Verification items for the finished model (mm, model axes). Face numbers are marked on the shaded views. A direction names the side the tool comes from. Give positions to 0.01 mm unless a question says otherwise; leave off trailing zeros. Write each loop counter-clockwise with the first axis right and the second up, starting at its lowest first coordinate (ties: lowest second). Pieces come first, ordered by that corner, then holes. Notation, with made-up numbers: (-11, -5.75) -> (19, -5.75) arc R22 ccw to (19, 33.25) -> close; hole circle Ø6 at (70, -11.5). An arc over 180 degrees is marked (long way). Use CSV: the item, a comma, the result in double quotes. Start each with the question number.
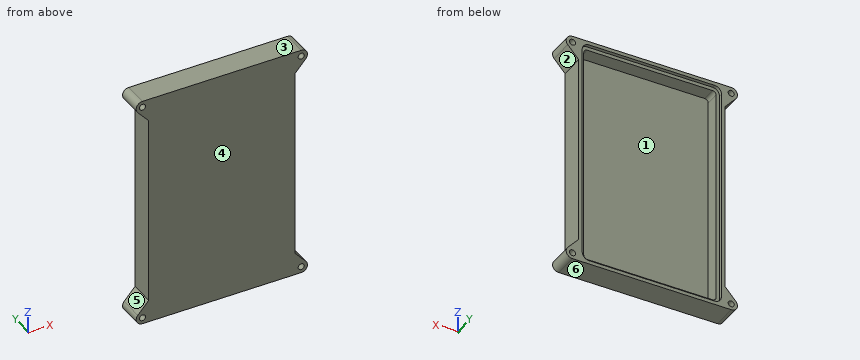
```python
from build123d import *

# Parameters (mm, degrees)
SALIENTE_EXTRUIR2_DEPTH   = 11
SALIENTE_EXTRUIR3_DEPTH   = 25.5
SALIENTE_EXTRUIR4_DEPTH   = 2.5
SALIENTE_EXTRUIR5_DEPTH   = 36.5
SIMETR_A2_COPY_1_DEPTH    = 36.5
CROQUIS6_R                = 2.2
CORTAR_EXTRUIR2_DEPTH     = 112.083302076
SIMETR_A4_COPY_1_SKETCH_R = 2.2
SIMETR_A4_COPY_1_DEPTH    = 112.083302076
CORTAR_EXTRUIR3_DEPTH     = 6
CORTAR_EXTRUIR4_START     = -18
CORTAR_EXTRUIR4_DEPTH     = 18
CORTAR_EXTRUIR5_START     = -13
CORTAR_EXTRUIR5_DEPTH     = 13


with BuildPart() as part:
    # Croquis1 → Saliente-Extruir2 (new body)
    # profile 1 of 3: a face of its own
    with BuildSketch(Plane(origin=(0, 0, 0), x_dir=(1, 0, 0), z_dir=(0, 1, 0))):
        with BuildLine():
            Line((-45, 85), (45, 85))
            ThreePointArc((45, 85), (50.303300859, 82.803300859), (52.5, 77.5))
            Line((52.5, 77.5), (52.5, -77.5))
            ThreePointArc((52.5, -77.5), (50.303300859, -82.803300859), (45, -85))
            Line((45, -85), (-45, -85))
            ThreePointArc((-45, -85), (-50.303300859, -82.803300859), (-52.5, -77.5))
            Line((-52.5, -77.5), (-52.5, 77.5))
            ThreePointArc((-52.5, 77.5), (-50.303300859, 82.803300859), (-45, 85))
        make_face()
        with BuildLine():
            ThreePointArc((-45, 82.5), (-48.535533906, 81.035533906), (-50, 77.5))
            Line((-50, 77.5), (-50, -77.5))
            ThreePointArc((-50, -77.5), (-48.535533906, -81.035533906), (-45, -82.5))
            Line((-45, -82.5), (45, -82.5))
            ThreePointArc((45, -82.5), (48.535533906, -81.035533906), (50, -77.5))
            Line((50, -77.5), (50, 77.5))
            ThreePointArc((50, 77.5), (48.535533906, 81.035533906), (45, 82.5))
            Line((45, 82.5), (-45, 82.5))
        make_face(mode=Mode.SUBTRACT)
    # profile 2 of 3: a face of its own
    with BuildSketch(Plane(origin=(0, 0, 0), x_dir=(1, 0, 0), z_dir=(0, 1, 0))):
        with BuildLine():
            Line((-45, 82.5), (45, 82.5))
            ThreePointArc((45, 82.5), (48.535533906, 81.035533906), (50, 77.5))
            Line((50, 77.5), (50, -77.5))
            ThreePointArc((50, -77.5), (48.535533906, -81.035533906), (45, -82.5))
            Line((45, -82.5), (-45, -82.5))
            ThreePointArc((-45, -82.5), (-48.535533906, -81.035533906), (-50, -77.5))
            Line((-50, -77.5), (-50, 77.5))
            ThreePointArc((-50, 77.5), (-48.535533906, 81.035533906), (-45, 82.5))
        make_face()
        with BuildLine():
            ThreePointArc((45, -80), (46.767766953, -79.267766953), (47.5, -77.5))
            Line((47.5, -77.5), (47.5, 77.5))
            ThreePointArc((47.5, 77.5), (46.767766953, 79.267766953), (45, 80))
            Line((45, 80), (-45, 80))
            ThreePointArc((-45, 80), (-46.767766953, 79.267766953), (-47.5, 77.5))
            Line((-47.5, 77.5), (-47.5, -77.5))
            ThreePointArc((-47.5, -77.5), (-46.767766953, -79.267766953), (-45, -80))
            Line((-45, -80), (45, -80))
        make_face(mode=Mode.SUBTRACT)
    # profile 3 of 3: a face of its own
    with BuildSketch(Plane(origin=(0, 0, 0), x_dir=(1, 0, 0), z_dir=(0, 1, 0))):
        with BuildLine():
            Line((-45, -80), (45, -80))
            ThreePointArc((45, -80), (46.767766953, -79.267766953), (47.5, -77.5))
            Line((47.5, -77.5), (47.5, 77.5))
            ThreePointArc((47.5, 77.5), (46.767766953, 79.267766953), (45, 80))
            Line((45, 80), (-45, 80))
            ThreePointArc((-45, 80), (-46.767766953, 79.267766953), (-47.5, 77.5))
            Line((-47.5, 77.5), (-47.5, -77.5))
            ThreePointArc((-47.5, -77.5), (-46.767766953, -79.267766953), (-45, -80))
        make_face()
    extrude(amount=SALIENTE_EXTRUIR2_DEPTH)

    # Croquis2 → Saliente-Extruir3 (add)
    # profile 1 of 2: a face of its own
    with BuildSketch(Plane(origin=(0, 11, 0), x_dir=(1, 0, 0), z_dir=(0, 1, 0))):
        with BuildLine():
            ThreePointArc((52.5, 77.5), (50.303300859, 82.803300859), (45, 85))
            Line((45, 85), (-45, 85))
            ThreePointArc((-45, 85), (-50.303300859, 82.803300859), (-52.5, 77.5))
            Line((-52.5, 77.5), (-52.5, -77.5))
            ThreePointArc((-52.5, -77.5), (-50.303300859, -82.803300859), (-45, -85))
            Line((-45, -85), (45, -85))
            ThreePointArc((45, -85), (50.303300859, -82.803300859), (52.5, -77.5))
            Line((52.5, -77.5), (52.5, 77.5))
        make_face()
        with BuildLine():
            ThreePointArc((-45, 82.5), (-48.535533906, 81.035533906), (-50, 77.5))
            Line((-50, 77.5), (-50, -77.5))
            ThreePointArc((-50, -77.5), (-48.535533906, -81.035533906), (-45, -82.5))
            Line((-45, -82.5), (45, -82.5))
            ThreePointArc((45, -82.5), (48.535533906, -81.035533906), (50, -77.5))
            Line((50, -77.5), (50, 77.5))
            ThreePointArc((50, 77.5), (48.535533906, 81.035533906), (45, 82.5))
            Line((45, 82.5), (-45, 82.5))
        make_face(mode=Mode.SUBTRACT)
    # profile 2 of 2: a face of its own
    with BuildSketch(Plane(origin=(0, 11, 0), x_dir=(1, 0, 0), z_dir=(0, 1, 0))):
        with BuildLine():
            Line((45, 82.5), (-45, 82.5))
            ThreePointArc((-45, 82.5), (-48.535533906, 81.035533906), (-50, 77.5))
            Line((-50, 77.5), (-50, -77.5))
            ThreePointArc((-50, -77.5), (-48.535533906, -81.035533906), (-45, -82.5))
            Line((-45, -82.5), (45, -82.5))
            ThreePointArc((45, -82.5), (48.535533906, -81.035533906), (50, -77.5))
            Line((50, -77.5), (50, 77.5))
            ThreePointArc((50, 77.5), (48.535533906, 81.035533906), (45, 82.5))
        make_face()
        with BuildLine():
            ThreePointArc((-45, 80), (-46.767766953, 79.267766953), (-47.5, 77.5))
            Line((-47.5, 77.5), (-47.5, -77.5))
            ThreePointArc((-47.5, -77.5), (-46.767766953, -79.267766953), (-45, -80))
            Line((-45, -80), (45, -80))
            ThreePointArc((45, -80), (46.767766953, -79.267766953), (47.5, -77.5))
            Line((47.5, -77.5), (47.5, 77.5))
            ThreePointArc((47.5, 77.5), (46.767766953, 79.267766953), (45, 80))
            Line((45, 80), (-45, 80))
        make_face(mode=Mode.SUBTRACT)
    extrude(amount=SALIENTE_EXTRUIR3_DEPTH)

    # Croquis3 → Saliente-Extruir4 (add)
    with BuildSketch(Plane(origin=(0, 36.5, 0), x_dir=(1, 0, 0), z_dir=(0, 1, 0))):
        with BuildLine():
            Line((45, 82.5), (-45, 82.5))
            ThreePointArc((-45, 82.5), (-48.535533906, 81.035533906), (-50, 77.5))
            Line((-50, 77.5), (-50, -77.5))
            ThreePointArc((-50, -77.5), (-48.535533906, -81.035533906), (-45, -82.5))
            Line((-45, -82.5), (45, -82.5))
            ThreePointArc((45, -82.5), (48.535533906, -81.035533906), (50, -77.5))
            Line((50, -77.5), (50, 77.5))
            ThreePointArc((50, 77.5), (48.535533906, 81.035533906), (45, 82.5))
        make_face()
        with BuildLine():
            Line((-47.5, -77.5), (-47.5, 77.5))
            ThreePointArc((-47.5, 77.5), (-46.767766953, 79.267766953), (-45, 80))
            Line((-45, 80), (45, 80))
            ThreePointArc((45, 80), (46.767766953, 79.267766953), (47.5, 77.5))
            Line((47.5, 77.5), (47.5, -77.5))
            ThreePointArc((47.5, -77.5), (46.767766953, -79.267766953), (45, -80))
            Line((45, -80), (-45, -80))
            ThreePointArc((-45, -80), (-46.767766953, -79.267766953), (-47.5, -77.5))
        make_face(mode=Mode.SUBTRACT)
    extrude(amount=SALIENTE_EXTRUIR4_DEPTH)

    # Croquis4 → Saliente-Extruir5 (add)
    with BuildSketch(Plane.XZ):
        with BuildLine():
            Line((57, 85), (45, 85))
            ThreePointArc((45, 85), (50.303300859, 82.803300859), (52.5, 77.5))
            Line((52.5, 77.5), (52.5, 68.686877301))
            Line((52.5, 68.686877301), (60.359510947, 77.506058418))
            ThreePointArc((60.359510947, 77.506058418), (61.10625968, 82.340823577), (57, 85))
        make_face()
    saliente_extruir5 = extrude(amount=-SALIENTE_EXTRUIR5_DEPTH)

    # Simetría1: Saliente-Extruir5 across plane
    add(saliente_extruir5.mirror(Plane(origin=(0, 0, 0), x_dir=(0, 0, 1), z_dir=(1, 0, 0))))

    # Simetría2: Saliente-Extruir5 across plane
    add(saliente_extruir5.mirror(Plane.XY))

    # Simetría2 copy 1 sketch → Simetría2 copy 1 (add)
    with BuildSketch(Plane(origin=(0, 0, 0), x_dir=(-1, 0, 0), z_dir=(0, -1, 0))):
        with BuildLine():
            Line((57, 85), (45, 85))
            ThreePointArc((45, 85), (50.303300859, 82.803300859), (52.5, 77.5))
            Line((52.5, 77.5), (52.5, 68.686877301))
            Line((52.5, 68.686877301), (60.359510947, 77.506058418))
            ThreePointArc((60.359510947, 77.506058418), (61.10625968, 82.340823577), (57, 85))
        make_face()
    extrude(amount=-SIMETR_A2_COPY_1_DEPTH)

    # Croquis6 → Cortar-Extruir2 (cut, through all)
    with BuildSketch(Plane(origin=(0, 36.5, 0), x_dir=(1, 0, 0), z_dir=(0, 1, 0))):
        with Locations(Location((57, 80.5, 0), (0, 0, 270))):
            Circle(CROQUIS6_R)
    cortar_extruir2 = extrude(amount=-CORTAR_EXTRUIR2_DEPTH, mode=Mode.SUBTRACT)

    # Simetría3: Cortar-Extruir2 across plane
    add(cortar_extruir2.mirror(Plane(origin=(0, 0, 0), x_dir=(0, 0, 1), z_dir=(1, 0, 0))), mode=Mode.SUBTRACT)

    # Simetría4: Cortar-Extruir2 across plane
    add(cortar_extruir2.mirror(Plane.XY), mode=Mode.SUBTRACT)

    # Simetría4 copy 1 sketch → Simetría4 copy 1 (cut, through all)
    with BuildSketch(Plane(origin=(0, 36.5, 0), x_dir=(-1, 0, 0), z_dir=(0, 1, 0))):
        with Locations(Location((57, 80.5, 0), (0, 0, 270))):
            Circle(SIMETR_A4_COPY_1_SKETCH_R)
    extrude(amount=-SIMETR_A4_COPY_1_DEPTH, mode=Mode.SUBTRACT)

    # Croquis8 → Cortar-Extruir3 (cut)
    with BuildSketch(Plane.XZ):
        with BuildLine():
            Line((-57, -85), (57, -85))
            ThreePointArc((57, -85), (61.10625968, -82.340823577), (60.359510947, -77.506058418))
            Line((60.359510947, -77.506058418), (52.5, -68.686877301))
            Line((52.5, -68.686877301), (52.5, 68.686877301))
            Line((52.5, 68.686877301), (60.359510947, 77.506058418))
            ThreePointArc((60.359510947, 77.506058418), (61.10625968, 82.340823577), (57, 85))
            Line((57, 85), (-57, 85))
            ThreePointArc((-57, 85), (-61.10625968, 82.340823577), (-60.359510947, 77.506058418))
            Line((-60.359510947, 77.506058418), (-52.5, 68.686877301))
            Line((-52.5, 68.686877301), (-52.5, -68.686877301))
            Line((-52.5, -68.686877301), (-60.359510947, -77.506058418))
            ThreePointArc((-60.359510947, -77.506058418), (-61.10625968, -82.340823577), (-57, -85))
        make_face()
    extrude(amount=-CORTAR_EXTRUIR3_DEPTH, mode=Mode.SUBTRACT)

    # Croquis9 → Cortar-Extruir4 (cut)
    with BuildSketch(Plane(origin=(0, 39, 0), x_dir=(1, 0, 0), z_dir=(0, 1, 0)).offset(CORTAR_EXTRUIR4_START)):
        with BuildLine():
            Line((45, 82.5), (-45, 82.5))
            ThreePointArc((-45, 82.5), (-48.535533906, 81.035533906), (-50, 77.5))
            Line((-50, 77.5), (-50, -77.5))
            ThreePointArc((-50, -77.5), (-48.535533906, -81.035533906), (-45, -82.5))
            Line((-45, -82.5), (45, -82.5))
            ThreePointArc((45, -82.5), (48.535533906, -81.035533906), (50, -77.5))
            Line((50, -77.5), (50, 77.5))
            ThreePointArc((50, 77.5), (48.535533906, 81.035533906), (45, 82.5))
        make_face()
        with BuildLine():
            Line((-47.5, 77.5), (-47.5, -77.5))
            ThreePointArc((-47.5, -77.5), (-46.767766953, -79.267766953), (-45, -80))
            Line((-45, -80), (45, -80))
            ThreePointArc((45, -80), (46.767766953, -79.267766953), (47.5, -77.5))
            Line((47.5, -77.5), (47.5, 77.5))
            ThreePointArc((47.5, 77.5), (46.767766953, 79.267766953), (45, 80))
            Line((45, 80), (-45, 80))
            ThreePointArc((-45, 80), (-46.767766953, 79.267766953), (-47.5, 77.5))
        make_face(mode=Mode.SUBTRACT)
    extrude(amount=CORTAR_EXTRUIR4_DEPTH, mode=Mode.SUBTRACT)

    # Croquis10 → Cortar-Extruir5 (cut)
    with BuildSketch(Plane(origin=(0, 36.5, 0), x_dir=(1, 0, 0), z_dir=(0, 1, 0)).offset(CORTAR_EXTRUIR5_START)):
        with BuildLine():
            Line((57, 85), (-57, 85))
            ThreePointArc((-57, 85), (-61.10625968, 82.340823577), (-60.359510947, 77.506058418))
            Line((-60.359510947, 77.506058418), (-52.5, 68.686877301))
            Line((-52.5, 68.686877301), (-52.5, -68.686877301))
            Line((-52.5, -68.686877301), (-60.359510947, -77.506058418))
            ThreePointArc((-60.359510947, -77.506058418), (-61.10625968, -82.340823577), (-57, -85))
            Line((-57, -85), (57, -85))
            ThreePointArc((57, -85), (61.10625968, -82.340823577), (60.359510947, -77.506058418))
            Line((60.359510947, -77.506058418), (52.5, -68.686877301))
            Line((52.5, -68.686877301), (52.5, 68.686877301))
            Line((52.5, 68.686877301), (60.359510947, 77.506058418))
            ThreePointArc((60.359510947, 77.506058418), (61.10625968, 82.340823577), (57, 85))
        make_face()
    extrude(amount=CORTAR_EXTRUIR5_DEPTH, mode=Mode.SUBTRACT)


solid = part.part
```
(1) Section check A-A on y = 9. Record the cut outline in (x, z), then the cut area to 3 significant figures.
(2) Section check D-D on x = -4. Record the cut outline in (y, z), then the cut area to 4 significant figures.
(3) Go/stop test with flat-tipped pins: pin 1 (1.5 mm diameter, centred on y = 15.5, z = 49, fed in from -X); pin 2 (0.8 mm diameter, centred on y = 22, z = 23, fed in from +X). Record where each tip stops, or that it passes through.
(4) Section check C-C on z = 57. Record the cut outline in (x, y), then the cut area to 4 significant figures.
(5) Section check B-B on y = 18.5. Record the cut outline in (x, z), then the cut area to 3 significant figures.
(6) Set-up check for the marked faces 5 and 6: record each of +Z, -Z, +X, -X, +Y, -Y from which the full face is reachable in a straight line by a thin tool's end or side.
(7) Draft check along Z on the marked faces 1, 2, 3 and 4. Enter one of: released by +Z, released by -Z, zero draft, split by the parting line, or undercut.
(8) Thickness scan on line 1 (X direction, y = 12.75, z = 80.5); line 2 (Z direction, x = 42, y = 22.25); line 3 (Z direction, x = -2.5, y = 19). Record the ranges inside material, lowest first. Write a range as from..to.
Data:
1,outline,"(-60.36, -77.51) arc R4.5 ccw to (-57, -85) -> (57, -85) arc R4.5 ccw to (60.36, -77.51) -> (52.5, -68.69) -> (52.5, 68.69) -> (60.36, 77.51) arc R4.5 ccw to (57, 85) -> (-57, 85) arc R4.5 ccw to (-60.36, 77.51) -> (-52.5, 68.69) -> (-52.5, -68.69) -> close; hole circle Ø4.4 at (-57, -80.5); hole circle Ø4.4 at (-57, 80.5); hole circle Ø4.4 at (57, -80.5); hole circle Ø4.4 at (57, 80.5)"
1,area,"18,200 mm2"
2,outline,"(6, -85) -> (23.5, -85) -> (23.5, -82.5) -> (21, -82.5) -> (21, -80) -> (11, -80) -> (11, 80) -> (21, 80) -> (21, 82.5) -> (23.5, 82.5) -> (23.5, 85) -> (6, 85) -> close"
2,area,"962.5 mm2"
3,pin 1,"stops at x = -52.5"
3,pin 2,"stops at x = 52.5"
4,outline,"(-52.5, 6) -> (52.5, 6) -> (52.5, 23.5) -> (50, 23.5) -> (50, 21) -> (47.5, 21) -> (47.5, 11) -> (-47.5, 11) -> (-47.5, 21) -> (-50, 21) -> (-50, 23.5) -> (-52.5, 23.5) -> close"
4,area,"637.5 mm2"
5,outline,"(-60.36, -77.51) arc R4.5 ccw to (-57, -85) -> (57, -85) arc R4.5 ccw to (60.36, -77.51) -> (52.5, -68.69) -> (52.5, 68.69) -> (60.36, 77.51) arc R4.5 ccw to (57, 85) -> (-57, 85) arc R4.5 ccw to (-60.36, 77.51) -> (-52.5, 68.69) -> (-52.5, -68.69) -> close; hole circle Ø4.4 at (-57, -80.5); hole circle Ø4.4 at (-57, 80.5); hole (-47.5, -77.5) arc R2.5 ccw to (-45, -80) -> (45, -80) arc R2.5 ccw to (47.5, -77.5) -> (47.5, 77.5) arc R2.5 ccw to (45, 80) -> (-45, 80) arc R2.5 ccw to (-47.5, 77.5) -> close; hole circle Ø4.4 at (57, -80.5); hole circle Ø4.4 at (57, 80.5)"
5,area,"2,980 mm2"
6,face 5,"-X, +Y, -Y"
6,face 6,"-Z, +X, -X, +Y, -Y"
7,face 1,"undercut"
7,face 2,"undercut"
7,face 3,"released by +Z"
7,face 4,"zero draft"
8,line 1,"x = -61.5..-59.2, -54.8..54.8, 59.2..61.5"
8,line 2,"z = -85..-82.5, 82.5..85"
8,line 3,"z = -85..-80, 80..85"
